Verification items for the finished model (mm, model axes). A direction names the side the tool comes from. Round coordinates to 2 decimals unless told otherwise and drop trailing zeros. Write each loop counter-clockwise with the first axis right and the second up, starting at its lowest first coordinate (ties: lowest second). Pieces come first, ordered by that corner, then holes. Notation, with made-up numbers: M 71.25,41.25 L 125.25,41.25 A21 cw 125.25,73.25 Z; hole C 8.5,51 d3. An arc over 180 degrees is marked long. One line per question, with ' | ' between items. Start each with the question number.
Q1. Cross-section at C-C (z = -13). Record the boundary of the cut face in (x, y).
Q2. Cross-section at B-B (x = -5). Record the boundary of the cut face in (y, z).
Q3. Gauge pin test, flat ends, axial feed: pin 1 (3 mm diameter, centred on y = -3, z = -9.5, fed in from +X); pin 2 (2 mm diameter, centred on x = 5, y = 4.5, fed in from +Z); pin 3 (2 mm diameter, centred on x = 5.5, y = -5, fed in from -Z). Record the tip position at first contact, or that the pin passes through.
Q4. Thickness scan on line 1 along Z through (x, y) = (2.75, -7); line 2 along Z through (x, y) = (-0.5, -5); line 3 along Y through (x, z) = (0.25, -4.75). Record the ranges inside material, lowest first. Write a range as from..to.
Q5. Tool access check on faces 1 (the face through (-3.796, 0.167, 3.779)), 2 (the face through (1.16, -5.223, -9.86)), 3 (the face through (-1.756, -7.907, 0.246)). Record the directions out of +Z, -Z, +X, -X, +Y, -Y that give a thin tool (end or side, any length) a straight path to the whole face; none if there is none.
Q6. Cross-section at A-A (y = 0). Record the boundary of the cut face in (x, z).
from build123d import *

# Parameters (mm, degrees)
ESQUISSE1_R        = 8.1
BOSS_EXTRU_1_DEPTH = 0.5
ESQUISSE2_R        = 5.9
BOSS_EXTRU_2_DEPTH = 1.8
ESQUISSE3_R        = 3.8
BOSS_EXTRU_3_DEPTH = 3
ESQUISSE4_R        = 5.35
BOSS_EXTRU_4_DEPTH = 20


with BuildPart() as part:
    # Esquisse1 → Boss.-Extru.1 (new body)
    with BuildSketch(Plane.XY):
        Circle(ESQUISSE1_R)
    extrude(amount=BOSS_EXTRU_1_DEPTH)

    # Esquisse2 → Boss.-Extru.2 (add)
    with BuildSketch(Plane.XY.offset(0.5)):
        Circle(ESQUISSE2_R)
    extrude(amount=BOSS_EXTRU_2_DEPTH)

    # Esquisse3 → Boss.-Extru.3 (add)
    with BuildSketch(Plane.XY.offset(2.3)):
        Circle(ESQUISSE3_R)
    extrude(amount=BOSS_EXTRU_3_DEPTH)

    # Esquisse4 → Boss.-Extru.4 (add)
    with BuildSketch(Plane(origin=(0, 0, 0), x_dir=(-1, 0, 0), z_dir=(0, 0, -1))):
        Circle(ESQUISSE4_R)
    extrude(amount=BOSS_EXTRU_4_DEPTH)


solid = part.part
Determined:
1) outline: C 0,0 d10.7
2) outline: M -6.37,0 L -1.9,0 L -1.9,-20 L 1.9,-20 L 1.9,0 L 6.37,0 L 6.37,0.5 L 3.13,0.5 L 3.13,2.3 L -3.13,2.3 L -3.13,0.5 L -6.37,0.5 Z
3) pin 1: stops at x = 5.14 | pin 2: stops at z = 2.3 | pin 3: stops at z = 0
4) line 1: z = 0..0.5 | line 2: z = -20..2.3 | line 3: y = -5.34..5.34
5) face 1: +Z | face 2: -Z | face 3: +Z, -Z
6) outline: M -8.1,0 L -5.35,0 L -5.35,-20 L 5.35,-20 L 5.35,0 L 8.1,0 L 8.1,0.5 L 5.9,0.5 L 5.9,2.3 L 3.8,2.3 L 3.8,5.3 L -3.8,5.3 L -3.8,2.3 L -5.9,2.3 L -5.9,0.5 L -8.1,0.5 Z
